Drawing for the job (mm, zero at the part's lowest x, y, z). A direction names the side the tool comes from. Give positions to 0.01 mm unless a question says otherwise; leave off trailing zeros. Write each loop counter-clockwise with the first axis right and the second up, starting at its lowest first coordinate (ties: lowest second). Pieces come first, ordered by that corner, then holes. Notation, with made-up numbers: M 54.5,-9 L 104.5,-9 A22 cw 104.5,4 Z; hole C -16.5,56 d4. An arc over 180 degrees is marked long. Answer as a JSON object with one key per item and string values. Group by question number.
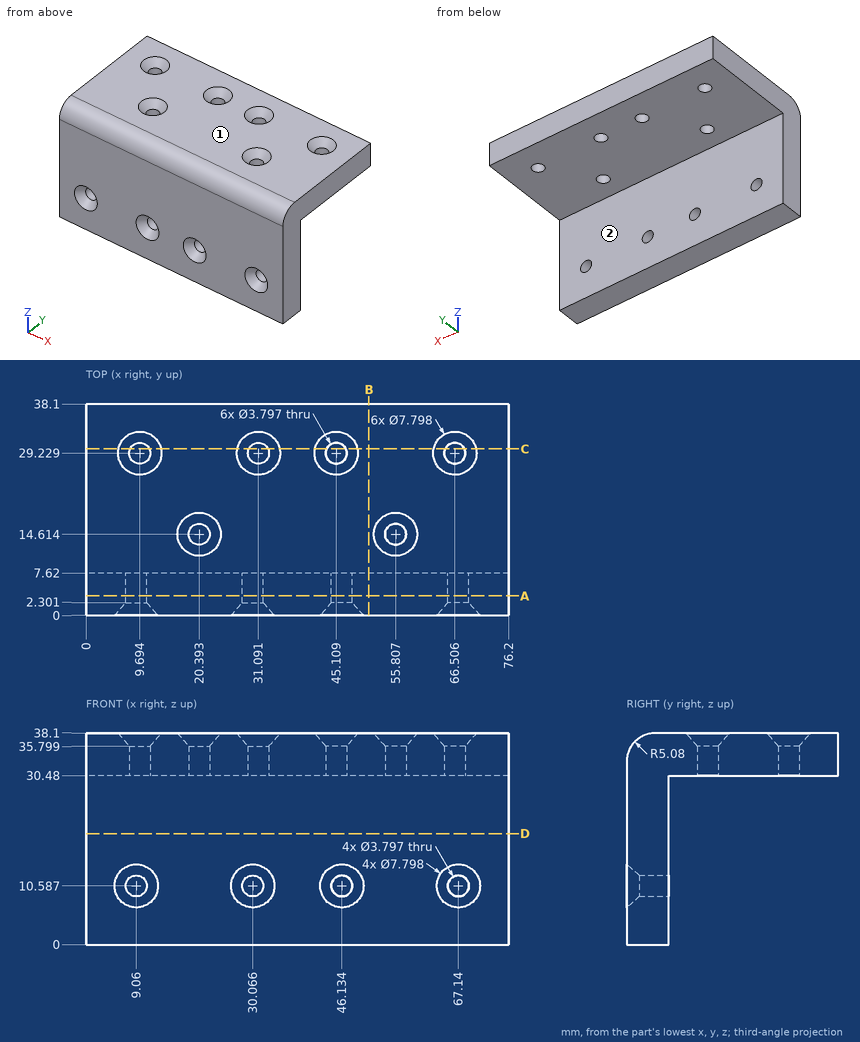
Q1. Slice it at C-C, the plane y = 30. Count the separate pieces of the cut face and the enclosed holes in it.
Q2. 3-axis set-ups, long thin cutter, end or side, ignore diameter. For the marked faces 1 and 2: which of +Z, -Z, +X, -X, +Y, -Y reach the whole face in a straight line?
Q3. Slice it at D-D, the plane z = 20. Write the cut outline in (x, y).
Q4. Slice it at A-A, the plane y = 3.5. Write the cut outline in (x, z) (1 decimal), then the cut area to 3 significant figures.
Q5. Drop flat-ended pins along their axis: P1, Ø5, axis at x = 65.5, y = 13, coming from the -Z side; P2, Ø6, axis at x = 28, z = 13, coming from the +Y side; P3, Ø3, axis at x = 20.39, y = 14.61, coming from the -Z side; P4, Ø5, axis at x = 55.81, y = 14.61, coming from the +Z side (1 decimal). Give the stop position or say it passes through.
Q6. Wall check: L1, parallel to Z at x = 19, y = 32.5; L2, parallel to Y at x = 9, z = 26.5; L3, parallel to Z at x = 29.5, y = 6.5 (1 decimal). Give the ranges that are in metal, low to high.
Q7. Slice it at B-B, the plane x = 51. Write the cut outline in (y, z), then the cut area to 3 significant figures.
Solved:
{
 "1": {"separate pieces": "5", "enclosed holes": "0"},
 "2": {"face 1": "+Z, +X, -X, +Y, -Y", "face 2": "-Z, +X, -X, +Y"},
 "3": {"outline": "M 0,0 L 76.2,0 L 76.2,7.62 L 0,7.62 Z"},
 "4": {"outline": "M 0,0 L 76.2,0 L 76.2,37.8 L 0,37.8 Z; hole C 9.1,10.6 d3.8; hole C 30.1,10.6 d3.8; hole C 46.1,10.6 d3.8; hole C 67.1,10.6 d3.8", "area": "2,840 mm²"},
 "5": {"P1": "stops at z = 30.48", "P2": "stops at y = 7.62", "P3": "passes through", "P4": "stops at z = 36.5"},
 "6": {"L1": "z = 30.48 to 38.1", "L2": "y = 0 to 7.62", "L3": "z = 0 to 8.8, 12.4 to 38.1"},
 "7": {"outline": "M 0,0 L 7.62,0 L 7.62,30.48 L 38.1,30.48 L 38.1,38.1 L 5.08,38.1 A5.08 ccw 0,33.02 Z", "area": "517 mm²"}
}
